Verification items for the finished model (mm, model axes). Face numbers are marked on the shaded views. A direction names the side the tool comes from. Give positions to 0.01 mm unless a question says otherwise; leave off trailing zeros. Loops run counter-clockwise (first coordinate to the right, second up) from the corner with the lowest first, then second, coordinate; pieces in that order, holes last. Notation, with made-up numbers: (14.5, 47.5) - (32.5, 47.5) arc R24 ccw to (32.5, 71.5) - close; hole circle Ø5 at (56.25, 66). An arc over 180 degrees is marked (long way). Answer in a Markdown table with one row per item.
```python
from build123d import *

# Parameters (mm, degrees)
ESQUISSE1_R                  = 18
ESQUISSE1_R_2                = 7.5
BOSS_EXTRU_1_DEPTH           = 45
ESQUISSE1_R_3                = 25
ESQUISSE1_R_4                = 12.5
BOSS_EXTRU_1_2_DEPTH         = 45
BOSS_EXTRU_2_START           = -3
BOSS_EXTRU_2_DEPTH           = 18
ESQUISSE4_R                  = 28
ESQUISSE4_R_2                = 16
BOSS_EXTRU_3_DEPTH           = 35
BOSS_EXTRU_4_DEPTH           = 31
ENL_V_MAT_EXTRU_1_DEPTH      = 201.129957777
ENL_V_MAT_EXTRU_1_DEPTH_BACK = 201.129957777
ESQUISSE6_W                  = 34
ESQUISSE6_H                  = 56
BOSS_EXTRU_5_DEPTH           = 21
BOSS_EXTRU_6_DEPTH           = 9
ESQUISSE10_W                 = 18
ESQUISSE10_H                 = 36
ENL_V_MAT_EXTRU_2_DEPTH      = 205.276773031


with BuildPart() as part:
    # Esquisse1 → Boss.-Extru.1 (new body)
    with BuildSketch(Plane(origin=(0, 0, 0), x_dir=(0, 0, -1), z_dir=(1, 0, 0))):
        with Locations(Location((0, 0, 0), (0, 0, 180))):
            Circle(ESQUISSE1_R)
        with Locations(Location((0, 0, 0), (0, 0, 180))):
            Circle(ESQUISSE1_R_2, mode=Mode.SUBTRACT)
    extrude(amount=BOSS_EXTRU_1_DEPTH)

    # Esquisse7 → Boss.-Extru.5 (add, symmetric)
    with BuildSketch(Plane.ZY.offset(-22.5)):
        with BuildLine():
            ThreePointArc((0, -18), (-18, 0), (0, 18))
            Line((0, 18), (-30, 18))
            Line((-30, 18), (-30, -18))
            Line((-30, -18), (0, -18))
        make_face()
    extrude(amount=BOSS_EXTRU_5_DEPTH, both=True)



with BuildPart() as body_2:
    # Esquisse1 → Boss.-Extru.1 2 (new body)
    with BuildSketch(Plane(origin=(0, 0, 0), x_dir=(0, 0, -1), z_dir=(1, 0, 0))):
        with Locations(Location((85, 0, 0), (0, 0, 180))):
            Circle(ESQUISSE1_R_3)
        with Locations(Location((85, 0, 0), (0, 0, 180))):
            Circle(ESQUISSE1_R_4, mode=Mode.SUBTRACT)
    extrude(amount=BOSS_EXTRU_1_2_DEPTH)

    # Esquisse3 → Boss.-Extru.2 (add)
    with BuildSketch(Plane(origin=(45, 0, 0), x_dir=(0, 0, -1), z_dir=(1, 0, 0)).offset(BOSS_EXTRU_2_START)):
        with BuildLine():
            Line((60, 0), (60, -70))
            Line((60, -70), (110, -70))
            Line((110, -70), (110, 0))
            ThreePointArc((110, 0), (85, -25), (60, 0))
        make_face()
    extrude(amount=-BOSS_EXTRU_2_DEPTH)



with BuildPart() as body_3:
    # Esquisse4 → Boss.-Extru.3 (new, symmetric)
    with BuildSketch(Plane(origin=(33, 0, 0), x_dir=(0, 0, -1), z_dir=(1, 0, 0))):
        with Locations((85, -110)):
            Circle(ESQUISSE4_R)
        with Locations((85, -110)):
            Circle(ESQUISSE4_R_2, mode=Mode.SUBTRACT)
    extrude(amount=BOSS_EXTRU_3_DEPTH, both=True)


with BuildPart() as body_2_1:
    add(body_2.part)

    add(body_3.part)  # Boss.-Extru.4 merges body 3
    # Esquisse5 → Boss.-Extru.4 (add, symmetric)
    with BuildSketch(Plane(origin=(33, 0, 0), x_dir=(0, 0, -1), z_dir=(1, 0, 0))):
        with BuildLine():
            Line((60, -70), (60, -97.390479787))
            ThreePointArc((60, -97.390479787), (85, -82), (110, -97.390479787))
            Line((110, -97.390479787), (110, -70))
            Line((110, -70), (60, -70))
        make_face()
    extrude(amount=BOSS_EXTRU_4_DEPTH, both=True)

    # Esquisse6 → Enl_v. mat.-Extru.1 (cut, two sides: drawn at the far end of the back side and taken through both)
    with BuildSketch(Plane(origin=(0, 0, -110), x_dir=(-1, 0, 0), z_dir=(0, 0, -1)).offset(-ENL_V_MAT_EXTRU_1_DEPTH_BACK)):
        with Locations((-33, -110)):
            Rectangle(ESQUISSE6_W, ESQUISSE6_H)
    extrude(amount=ENL_V_MAT_EXTRU_1_DEPTH + ENL_V_MAT_EXTRU_1_DEPTH_BACK, mode=Mode.SUBTRACT)


with BuildPart() as part_1:
    add(part.part)

    add(body_2_1.part)  # Boss.-Extru.6 merges body 2
    # Esquisse7_4 → Boss.-Extru.6 (add, symmetric)
    with BuildSketch(Plane.ZY.offset(-22.5)):
        with BuildLine():
            Line((-30, -18), (-30, 18))
            Line((-30, 18), (-67.650648427, 18))
            ThreePointArc((-67.650648427, 18), (-60, 0), (-67.650648427, -18))
            Line((-67.650648427, -18), (-30, -18))
        make_face()
    extrude(amount=BOSS_EXTRU_6_DEPTH, both=True)

    # Esquisse10 → Enl_v. mat.-Extru.2 (cut, through all)
    with BuildSketch(Plane(origin=(0, 18, 0), x_dir=(1, 0, 0), z_dir=(0, 1, 0))):
        with Locations((21, 0)):
            Rectangle(ESQUISSE10_W, ESQUISSE10_H)
    extrude(amount=-ENL_V_MAT_EXTRU_2_DEPTH, mode=Mode.SUBTRACT)


solid = part_1.part
```
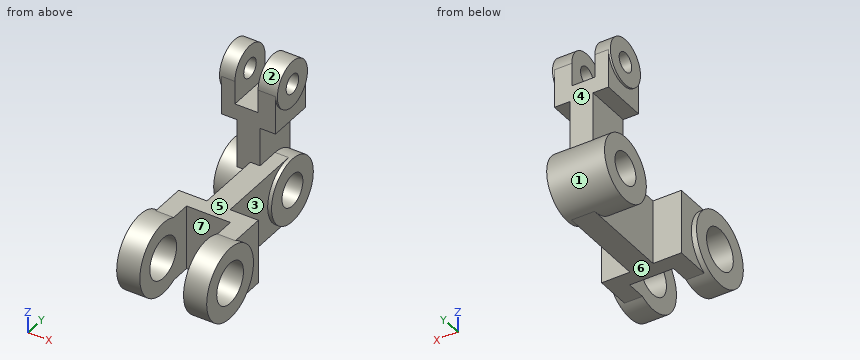
Q1. Sectioned sample at C-C (x = 19). Record the cut outline in (y, z).
Completed:
| item | result |
|---|---|
| outline | (-82, -110) - (-70, -110) - (-70, -60) - (-82, -60) - close; (-18, -67.65) arc R25 ccw (long way) to (18, -67.65) - (18, -18) - (-18, -18) - close; hole circle Ø25 at (0, -85) |
Q2. Thickness scan on line 1 (Y direction, x = 59, z = -85); line 2 (Z direction, x = 6, y = -110); line 3 (Y direction, x = 64.25, z = -85). Record the ranges inside material, lowest first.
Completed:
| item | result |
|---|---|
| line 1 | -138 to -126, -94 to -70 |
| line 2 | -113 to -101, -69 to -57 |
| line 3 | -138 to -126, -94 to -82 |
Q3. Sectioned sample at B-B (y = -110). Record the cut outline in (x, z).
Completed:
| item | result |
|---|---|
| outline | (-2, -113) - (16, -113) - (16, -101) - (-2, -101) - close; (-2, -69) - (16, -69) - (16, -57) - (-2, -57) - close; (50, -113) - (68, -113) - (68, -101) - (50, -101) - close; (50, -69) - (68, -69) - (68, -57) - (50, -57) - close |
Q4. Sectioned sample at D-D (z = -85). Give the number of separate pieces and of enclosed holes in the cut face, and give its area (3 significant figures).
Completed:
| item | result |
|---|---|
| separate pieces | 4 |
| enclosed holes | 0 |
| area | 3,540 mm^2 |
Q5. Draft check along Y on the marked faces 1, 2, 3 and 4. Enter one of: +Y half, -Y half, draft (parallel to the pull), parting line (faces both ways), or undercut.
Completed:
| item | result |
|---|---|
| face 1 | undercut |
| face 2 | parting line |
| face 3 | undercut |
| face 4 | +Y half |
Q6. Tool access check on the marked faces 5, 6 and 7. Record the directions out of +Z, -Z, +X, -X, +Y, -Y that give a thin tool (end or side, any length) a straight path to the whole face; none if there is none.
Completed:
| item | result |
|---|---|
| face 5 | +X |
| face 6 | -Z, +X, -X, +Y |
| face 7 | +Z, -Z, -Y |
Q7. Go/stop test with flat-tipped pins: P1, Ø15, axis at y = -8.5, z = -95, coming from the -X side; P2, Ø13, axis at x = 10.5, y = -8.5, coming from the -Z side; P3, Ø1, axis at x = 33, y = -75, coming from the -Z side. Record where each tip stops, or that it passes through.
Completed:
| item | result |
|---|---|
| P1 | x = 0 |
| P2 | z = -109.92 |
| P3 | z = -110 |
Q8. Sectioned sample at A-A (x = 34). Record the cut outline in (y, z).
Completed:
| item | result |
|---|---|
| outline | (-82, -110) - (0, -110) arc R25 ccw to (0, -60) - (-82, -60) - close; (-18, -30) - (18, -30) - (18, 0) arc R18 ccw to (-18, 0) - close; hole circle Ø25 at (0, -85); hole circle Ø15 at (0, 0) |
